Geometry: final body of the model. Coordinates: model frame, mm. A direction names the side the tool comes from. Give positions to 0.01 mm unless a question says otherwise; leave off trailing zeros. Order: outer loops, then holes, each group sorted by start corner. A loop starts at its lowest first (then second) coordinate and runs counter-clockwise, first axis right, second up. Notation, with made-up numbers: (-3.5, 50) -> (11.5, 50) arc R16 cw to (11.5, 59) -> close; hole circle Ø10 at (15.5, -33). An arc over 180 degrees is marked (long way). Answer in a Markdown table with one row per item. Add a question column.
Q1. Line query: line 1 along X through (y, z) = (-7.5, -6.5) (3 decimals); line 2 along Z through (x, y) = (0.75, 7.5) (3 decimals); line 3 along Z through (x, y) = (4, -10). Output: solid intervals per line, ascending. Write a range as from..to.
Q2. Set-up query: faces 4 (the face through (-3.175, 0, -2)), 5 (the face through (3, 8.063, -2)), 6 (the face through (3, -8.057, -2)), 7 (the face through (3, 0, -3.175)). Return all of +Z, -Z, +X, -X, +Y, -Y with unobstructed straight access to the full face (end or side cutting, diameter ignored); none if empty.
Q3. Cut plane D-D on x = -3.5. Return the cut outline in (y, z), and give its area (3 significant figures).
Q4. Contact query for flat-ended pins moving along their axis: P1, Ø4, axis at x = 7.5, y = -6.5, coming from the -Z side (3 decimals); P2, Ø5, axis at y = 2.5, z = -9.5, coming from the +X side; P3, Ø1.7, axis at x = 4.5, z = -2.5, coming from the +Y side. Output: stop coordinate, or through.
Q5. Cut plane A-A on x = 2.5. Return the cut outline in (y, z) (1 decimal), and give its area (3 significant figures).
Q6. Pull-direction query (X, two-part tool) for faces 1 (the face through (-4, 0, -1.588)), 2 (the face through (-8, 0, -12.7)), 3 (the face through (9.525, 0, -2)); classes: +X half, -X half, draft (parallel to the pull), parting line (faces both ways), or undercut.
from build123d import *

# Parameters (mm, degrees)
F0_W     = 12.7
F0_H     = 3.0555259615
F0_H_2   = 3.0494434938
F1_DEPTH = 1.5875
F0_W_2   = 3.175
F0_H_3   = 22.225
F2_DEPTH = 12.7
F0_H_4   = 16.1200305447
F3_DEPTH = 3.175


with BuildPart() as f1:
    # F0 (on Top) → F1 (new body)
    with BuildSketch(Plane.XY):
        Polygon((-3.175, 8.0630565062), (-3.175, 11.1125), (-6.35, 11.1125), (-6.35, -11.1125), (-3.175, -11.1125), (-3.175, -8.0569740385), align=None)
        with Locations((3.175, -9.5847370192)):
            Rectangle(F0_W, F0_H)
        with Locations((3.175, 9.5877782531)):
            Rectangle(F0_W, F0_H_2)
    extrude(amount=-F1_DEPTH)

    # F0 (on Top) → F2 (join)
    with BuildSketch(Plane.XY):
        with Locations((-7.9375, 0)):
            Rectangle(F0_W_2, F0_H_3)
    extrude(amount=-F2_DEPTH)

    # F0 (on Top) → F3 (join)
    with BuildSketch(Plane.XY):
        with Locations((3.175, 0.0030412339)):
            Rectangle(F0_W, F0_H_4)
    extrude(amount=-F3_DEPTH)


solid = f1.part
Completed:
| question | item | result |
|---|---|---|
| 1 | line 1 | x = -9.525..-6.35 |
| 1 | line 2 | z = -3.175..0 |
| 1 | line 3 | z = -1.59..0 |
| 2 | face 4 | -Z, +Y, -Y |
| 2 | face 5 | -Z, +X, +Y |
| 2 | face 6 | -Z, +X, -Y |
| 2 | face 7 | -Z, +X, +Y, -Y |
| 3 | outline | (-11.11, -1.59) -> (11.11, -1.59) -> (11.11, 0) -> (-11.11, 0) -> close |
| 3 | area | 35.3 mm² |
| 4 | P1 | stops at z = -3.175 |
| 4 | P2 | stops at x = -6.35 |
| 4 | P3 | stops at y = 8.06 |
| 5 | outline | (-11.1, -1.6) -> (-8.1, -1.6) -> (-8.1, -3.2) -> (8.1, -3.2) -> (8.1, -1.6) -> (11.1, -1.6) -> (11.1, 0) -> (-11.1, 0) -> close |
| 5 | area | 60.9 mm² |
| 6 | face 1 | undercut |
| 6 | face 2 | draft |
| 6 | face 3 | +X half |
